The model under review builds one solid part; all positions refer to its coordinate system, in mm. Coordinates: 2 decimals unless noted, no trailing zeros. Loops run counter-clockwise (first coordinate to the right, second up) from the corner with the lowest first, then second, coordinate; pieces in that order, holes last. Notation, with made-up numbers: M 17.25,34 L 22.25,34 A27 ccw 22.25,63 Z; hole C 28,79 d6. An arc over 180 degrees is marked long. Use CSV: the item, a comma, the result in double quotes. Start each with the question number.
1. For L1, parallel to Y at x = -42.75, z = 90; L2, parallel to X at y = -73.5, z = 411.5; L3, parallel to X at y = -61.5, z = 424.5, list the stretches that pass through material, from the lowest coordinate up.
2. Add section B-B, the plane y = -71.75. Write out the cut boundary in (x, z).
3. Add section A-A, the plane z = 160. Write out the cut boundary in (x, y).
4. Clearance check with flat-ended pins moving along their axes: P1, Ø1, axis at x = -27, z = 136, coming from the -Y side; P2, Ø2, axis at y = -71, z = 410.5, coming from the +X side; P3, Ø2, axis at x = -36.5, z = 120.5, coming from the -Y side. State where each tip first meets the part, or that it passes through.
5. Add section C-C, the plane x = -31.5. Write out the cut boundary in (y, z), then the cut area to 3 significant figures.
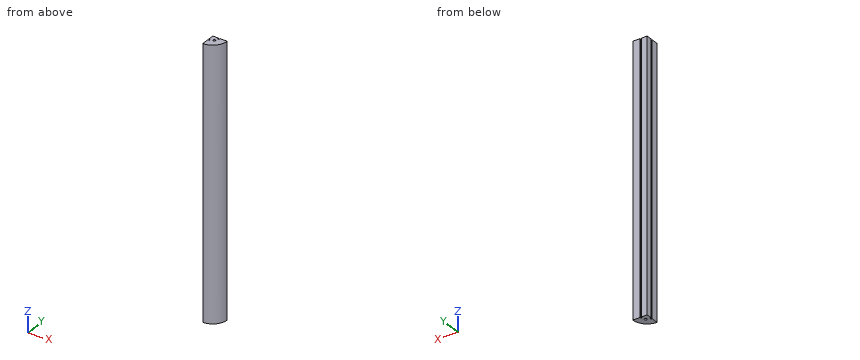
from build123d import *

# Parameters (mm, degrees)
F0_R     = 2.5
F1_DEPTH = 560


with BuildPart() as f1:
    # F0 (on Top) → F1 (new body)
    with BuildSketch(Plane.XY):
        with BuildLine():
            Line((-40.643933, -50.164693), (-52.643933, -50.164693))
            Line((-52.643933, -50.164693), (-52.643933, -62.164693))
            Line((-52.643933, -62.164693), (-49.643933, -62.164693))
            Line((-49.643933, -62.164693), (-49.643933, -65.164693))
            Line((-49.643933, -65.164693), (-52.643933, -65.164693))
            Line((-52.643933, -65.164693), (-52.643933, -80.164693))
            ThreePointArc((-52.643933, -80.164693), (-31.43073, -71.377897), (-22.643933, -50.164693))
            Line((-22.643933, -50.164693), (-37.643933, -50.164693))
            Line((-37.643933, -50.164693), (-37.643933, -53.164693))
            Line((-37.643933, -53.164693), (-40.643933, -53.164693))
            Line((-40.643933, -53.164693), (-40.643933, -50.164693))
        make_face()
        with Locations((-42.264516, -60.54411)):
            Circle(F0_R, mode=Mode.SUBTRACT)
    extrude(amount=F1_DEPTH)


solid = f1.part
Computed:
1,L1,"y = -78.49 to -63, -58.09 to -50.16"
1,L2,"x = -52.64 to -33.79"
1,L3,"x = -52.64 to -44.57, -39.95 to -24.87"
2,outline,"M -52.64,0 L -31.81,0 L -31.81,560 L -52.64,560 Z"
3,outline,"M -52.64,-80.16 A30 ccw -22.64,-50.16 L -37.64,-50.16 L -37.64,-53.16 L -40.64,-53.16 L -40.64,-50.16 L -52.64,-50.16 L -52.64,-62.16 L -49.64,-62.16 L -49.64,-65.16 L -52.64,-65.16 Z; hole C -42.26,-60.54 d5"
4,P1,"stops at y = -66.53"
4,P2,"stops at x = -30.14"
4,P3,"stops at y = -76.06"
5,outline,"M -71.45,0 L -50.16,0 L -50.16,560 L -71.45,560 Z"
5,area,"11,900 mm^2"
